from build123d import *

# Parameters (mm, degrees)
SKETCH_1_W                   = 65
SKETCH_1_H                   = 55
EXTRUDE_1_DEPTH              = 3
FILLET_1_R                   = 2
SKETCH_2_R                   = 1.525
CUT_EXTRUDE_1_DEPTH          = 6
HOLE_WIZARD_M3_1_D           = 3
HOLE_WIZARD_M3_1_DEPTH       = 7.25
HOLE_WIZARD_M3_1_CSINK_D     = 6.6
HOLE_WIZARD_M3_1_CSINK_ANGLE = 90
HOLE_WIZARD_M3_1_TIP         = 0.901290929
SKETCH_9_R                   = 1.5
CUT_EXTRUDE_3_DEPTH          = 10
SKETCH_13_W                  = 49
SKETCH_13_H                  = 31
CUT_EXTRUDE_8_DEPTH          = 10
FILLET_5_R                   = 2


with BuildPart() as part:
    # 草图1 → 凸台-拉伸1 (new body)
    with BuildSketch(Plane.XY):
        Rectangle(SKETCH_1_W, SKETCH_1_H)
    extrude(amount=EXTRUDE_1_DEPTH)

    # 圆角1
    fillet_1_edges = [part.edges().sort_by_distance(p)[0] for p in [
        (32.5, -27.5, 1.5),
        (-32.5, -27.5, 1.5),
        (-32.5, 27.5, 1.5),
        (32.5, 27.5, 1.5),
    ]]
    fillet(fillet_1_edges, radius=FILLET_1_R)

    # 草图2 → 切除-拉伸1 (cut)
    with BuildSketch(Plane(origin=(0, 0, 0), x_dir=(-1, 0, 0), z_dir=(0, 0, -1))):
        with Locations((20, -18.5)):
            Circle(SKETCH_2_R)
        with Locations((20, 18.5)):
            Circle(SKETCH_2_R)
    extrude(amount=-CUT_EXTRUDE_1_DEPTH, mode=Mode.SUBTRACT)

    # M3 十字槽沉头木螺钉的锥形沉头孔1
    with Locations(Plane(origin=(0, 0, 0), x_dir=(-1, 0, 0), z_dir=(0, 0, -1))):
        with Locations((20, 18.5)):
            CounterSinkHole(HOLE_WIZARD_M3_1_D / 2, HOLE_WIZARD_M3_1_CSINK_D / 2, depth=HOLE_WIZARD_M3_1_DEPTH, counter_sink_angle=HOLE_WIZARD_M3_1_CSINK_ANGLE)
            with Locations((0, 0, -(HOLE_WIZARD_M3_1_DEPTH + HOLE_WIZARD_M3_1_TIP / 2))):  # 118° drill point
                Cone(0, HOLE_WIZARD_M3_1_D / 2, HOLE_WIZARD_M3_1_TIP, mode=Mode.SUBTRACT)

    # 草图9 → 切除-拉伸3 (cut)
    with BuildSketch(Plane(origin=(0, 0, 0), x_dir=(-1, 0, 0), z_dir=(0, 0, -1))):
        with Locations((-12.5, 20)):
            Circle(SKETCH_9_R)
        with Locations((-12.5, -20)):
            Circle(SKETCH_9_R)
    extrude(amount=-CUT_EXTRUDE_3_DEPTH, mode=Mode.SUBTRACT)

    # 草图13 → 切除-拉伸8 (cut)
    with BuildSketch(Plane(origin=(0, 0, 0), x_dir=(-1, 0, 0), z_dir=(0, 0, -1))):
        Rectangle(SKETCH_13_W, SKETCH_13_H)
    extrude(amount=-CUT_EXTRUDE_8_DEPTH, mode=Mode.SUBTRACT)

    # 圆角5
    fillet_5_edges = [part.edges().sort_by_distance(p)[0] for p in [
        (-24.5, 15.5, 1.5),
        (-24.5, -15.5, 1.5),
        (24.5, -15.5, 1.5),
        (24.5, 15.5, 1.5),
    ]]
    fillet(fillet_5_edges, radius=FILLET_5_R)


solid = part.part
Part model, mm, in its own coordinate system. A direction names the side the tool comes from. Give positions to 0.01 mm unless a question says otherwise; leave off trailing zeros. Loops run counter-clockwise (first coordinate to the right, second up) from the corner with the lowest first, then second, coordinate; pieces in that order, holes last.
(1) Band-saw the part on B-B (x = -13.5). Write the cut outline in (y, z).
Return value:
outline: (-27.5, 0) - (-15.5, 0) - (-15.5, 3) - (-27.5, 3) - close; (15.5, 0) - (27.5, 0) - (27.5, 3) - (15.5, 3) - close
(2) 3-axis set-ups, long thin cutter, end or side, ignore diameter. For faces 1 (the flat face through (24.5, 0, 1)), 2 (the flat face through (0, 27.5, 1)): which of +Z, -Z, +X, -X, +Y, -Y reach the whole face in a straight line?
Return value:
face 1: +Z, -Z
face 2: +Z, -Z, +X, -X, +Y
(3) Drill centre lines: line 1 along Y through (x, z) = (-20, 2.15) (3 decimals); line 2 along Y through (x, z) = (2, 1.25); line 3 along X through (y, z) = (-13.5, 2.1). Where is each one in solid material? Low to high.
Return value:
line 1: y = -27.5 to -20.025, -16.975 to -15.5, 15.5 to 16.975, 20.025 to 27.5
line 2: y = -27.5 to -15.5, 15.5 to 27.5
line 3: x = -32.5 to -24.5, 24.5 to 32.5
(4) Band-saw the part on C-C (x = -20). Write the cut outline in (y, z) (3 decimals), and give its area (3 significant figures).
Return value:
outline: (-27.5, 0) - (-20.025, 0) - (-20.025, 3) - (-27.5, 3) - close; (-16.975, 0) - (-15.5, 0) - (-15.5, 3) - (-16.975, 3) - close; (15.5, 0.3) - (16.975, 1.775) - (16.975, 3) - (15.5, 3) - close; (20.025, 1.775) - (21.8, 0) - (27.5, 0) - (27.5, 3) - (20.025, 3) - close
area: 50.6 mm2
(5) Band-saw the part on A-A (y = 0.5). Write the cut outline in (x, z), and give its area (3 significant figures).
Return value:
outline: (-32.5, 0) - (-24.5, 0) - (-24.5, 3) - (-32.5, 3) - close; (24.5, 0) - (32.5, 0) - (32.5, 3) - (24.5, 3) - close
area: 48.0 mm2
(6) Pull direction X, two halves, no side cores. Call faces 3 (the cylindrical face through (31.93, 26.9, 1.52)), 4 (the flat face through (0, 19, 3)), 5 (the cylindrical face through (-23.93, -14.9, 1.52)): pulls with the +X half, pulls with the -X half, needs draft (parallel to the pull), parting line crosses it, or undercut.
Return value:
face 3: pulls with the +X half
face 4: needs draft
face 5: undercut
